Here's how the part is built. I have some questions about the finished solid (model axes, mm). Face numbers are marked on the shaded views. A direction names the side the tool comes from. Round coordinates to 2 decimals unless told otherwise and drop trailing zeros. Order: outer loops, then holes, each group sorted by start corner. A loop starts at its lowest first (then second) coordinate and runs counter-clockwise, first axis right, second up. Notation, with made-up numbers: (18.25, 35.25) -> (66.25, 35.25) arc R29 ccw to (66.25, 74.25) -> close; hole circle Ø7 at (48.25, 61). An arc over 180 degrees is marked (long way). Answer in a Markdown table with one row per item.
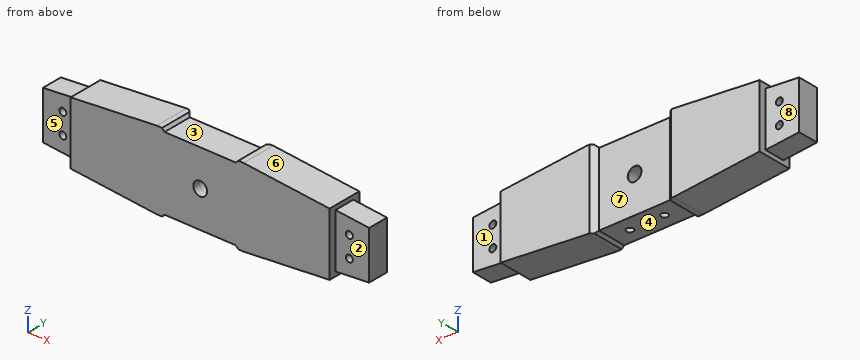
```python
from build123d import *

# Parameters (mm, degrees)
SKETCH1_R                = 4
BOSS_EXTRUDE1_DEPTH      = 12
SKETCH2_R                = 4
BOSS_EXTRUDE2_DEPTH      = 4
BOSS_EXTRUDE2_DEPTH_BACK = 16
CUT_EXTRUDE1_DEPTH       = 1
CUT_EXTRUDE1_DEPTH_BACK  = 46
SKETCH6_R                = 2.05
CUT_EXTRUDE3_DEPTH       = 6.5
SKETCH7_R                = 2
CUT_EXTRUDE4_DEPTH       = 17
CUT_EXTRUDE5_DEPTH       = 1
CUT_EXTRUDE5_DEPTH_BACK  = 21
CUT_EXTRUDE6_DEPTH       = 17


with BuildPart() as part:
    # Sketch1 → Boss-Extrude1 (new body)
    with BuildSketch(Plane(origin=(0, 0, 0), x_dir=(1, 0, 0), z_dir=(0, 1, 0))):
        Polygon((25, 20), (-25, 20), (-95, 13.834935185), (-95, -13.834935185), (-25, -20), (25, -20), (95, -13.834935185), (95, 13.834935185), align=None)
        Circle(SKETCH1_R, mode=Mode.SUBTRACT)
    extrude(amount=BOSS_EXTRUDE1_DEPTH)

    # Sketch2 → Boss-Extrude2 (add, two sides)
    with BuildSketch(Plane(origin=(0, 12, 0), x_dir=(1, 0, 0), z_dir=(0, 1, 0))) as boss_extrude2_sk:
        Polygon((-25, 20), (-75, 15.596382275), (-75, -15.596382275), (-25, -20), (25, -20), (75, -15.596382275), (75, 15.596382275), (25, 20), align=None)
        Circle(SKETCH2_R, mode=Mode.SUBTRACT)
        Polygon((-25, -20), (-75, -15.596382275), (-75, -18.10605947), (-25.109877781, -22.5), (25.109877781, -22.5), (75, -18.10605947), (75, -15.596382275), (25, -20), align=None)
        Polygon((-25.109877781, 22.5), (-75, 18.10605947), (-75, 15.596382275), (-25, 20), (25, 20), (75, 15.596382275), (75, 18.10605947), (25.109877781, 22.5), align=None)
    extrude(amount=BOSS_EXTRUDE2_DEPTH)
    extrude(boss_extrude2_sk.sketch, amount=-BOSS_EXTRUDE2_DEPTH_BACK)

    # Sketch3 → Cut-Extrude1 (cut, two sides)
    with BuildSketch(Plane.XY.offset(22.5)) as cut_extrude1_sk:
        Polygon((23.609877781, 16), (-23.609877781, 16), (-20.609877781, 13), (20.609877781, 13), align=None)
    extrude(amount=CUT_EXTRUDE1_DEPTH, mode=Mode.SUBTRACT)
    extrude(cut_extrude1_sk.sketch, amount=-CUT_EXTRUDE1_DEPTH_BACK, mode=Mode.SUBTRACT)

    # Sketch6 → Cut-Extrude3 (cut)
    with BuildSketch(Plane(origin=(0, 0, -22.5), x_dir=(-1, 0, 0), z_dir=(0, 0, -1))):
        with Locations((-10, 4.5)):
            Circle(SKETCH6_R)
        with Locations((10, 4.5)):
            Circle(SKETCH6_R)
    extrude(amount=-CUT_EXTRUDE3_DEPTH, mode=Mode.SUBTRACT)

    # Sketch7 → Cut-Extrude4 (cut, through all)
    with BuildSketch(Plane.XZ):
        with Locations((-83, -6)):
            Circle(SKETCH7_R)
        with Locations((-83, 6)):
            Circle(SKETCH7_R)
        with Locations((83, 6)):
            Circle(SKETCH7_R)
        with Locations((83, -6)):
            Circle(SKETCH7_R)
    extrude(amount=-CUT_EXTRUDE4_DEPTH, mode=Mode.SUBTRACT)

    # Sketch8 → Cut-Extrude5 (cut, two sides)
    with BuildSketch(Plane.XZ.offset(4)) as cut_extrude5_sk:
        Polygon((-22.109877781, -22.5), (-20.609877781, -21), (20.609877781, -21), (22.109877781, -22.5), align=None)
        Polygon((-22.109877781, 22.5), (22.109877781, 22.5), (20.609877781, 21), (-20.609877781, 21), align=None)
    extrude(amount=CUT_EXTRUDE5_DEPTH, mode=Mode.SUBTRACT)
    extrude(cut_extrude5_sk.sketch, amount=-CUT_EXTRUDE5_DEPTH_BACK, mode=Mode.SUBTRACT)

    # Sketch9 → Cut-Extrude6 (cut, through all)
    with BuildSketch(Plane(origin=(0, 12, 0), x_dir=(1, 0, 0), z_dir=(0, 1, 0))):
        Polygon((-94.5, 13.878971362), (-94.5, -13.878971362), (-95, -13.834935185), (-95, 13.834935185), align=None)
        Polygon((94.5, 13.878971362), (94.5, -13.878971362), (95, -13.834935185), (95, 13.834935185), align=None)
    extrude(amount=-CUT_EXTRUDE6_DEPTH, mode=Mode.SUBTRACT)


solid = part.part
```
1. Suppose I cut it at A-A on z = -6. Write out the boundary of the cut face in (x, y).
Numbers:
| item | result |
|---|---|
| outline | (-94.5, 0) -> (-85, 0) -> (-85, 12) -> (-94.5, 12) -> close; (-81, 0) -> (-75, 0) -> (-75, -4) -> (75, -4) -> (75, 0) -> (81, 0) -> (81, 12) -> (75, 12) -> (75, 16) -> (23.61, 16) -> (20.61, 13) -> (-20.61, 13) -> (-23.61, 16) -> (-75, 16) -> (-75, 12) -> (-81, 12) -> close; (85, 0) -> (94.5, 0) -> (94.5, 12) -> (85, 12) -> close |
2. Suppose I cut it at C-C on z = 10. Write out the boundary of the cut face in (x, y), then the cut area to 3 significant figures.
Numbers:
| item | result |
|---|---|
| outline | (-94.5, 0) -> (-75, 0) -> (-75, -4) -> (75, -4) -> (75, 0) -> (94.5, 0) -> (94.5, 12) -> (75, 12) -> (75, 16) -> (23.61, 16) -> (20.61, 13) -> (-20.61, 13) -> (-23.61, 16) -> (-75, 16) -> (-75, 12) -> (-94.5, 12) -> close |
| area | 3,340 mm2 |
3. Suppose I cut it at D-D on x = -83. Write out the boundary of the cut face in (y, z), then the cut area to 3 significant figures.
Numbers:
| item | result |
|---|---|
| outline | (0, -14.89) -> (12, -14.89) -> (12, -8) -> (0, -8) -> close; (0, -4) -> (12, -4) -> (12, 4) -> (0, 4) -> close; (0, 8) -> (12, 8) -> (12, 14.89) -> (0, 14.89) -> close |
| area | 261 mm2 |
4. We'd pull the mould along X, two halves only. Please class the marked faces 6, 7 and 8: released by +X, released by -X, zero draft, split by the parting line, or undercut.
Numbers:
| item | result |
|---|---|
| face 6 | released by +X |
| face 7 | undercut |
| face 8 | zero draft |
5. Please list where these lines run through material, in increasing order: line 1 along Y through (x, z) = (10, -19.3); line 2 along Z through (x, y) = (0, -2.95); line 3 along X through (y, z) = (-2.9, 0).
Numbers:
| item | result |
|---|---|
| line 1 | y = -4 to 2.45, 6.55 to 13 |
| line 2 | z = -21 to -4, 4 to 21 |
| line 3 | x = -75 to -4, 4 to 75 |
6. Suppose I cut it at B-B on x = 0. Write out the boundary of the cut face in (y, z), then the cut area to 3 significant figures.
Numbers:
| item | result |
|---|---|
| outline | (-4, -21) -> (13, -21) -> (13, -4) -> (-4, -4) -> close; (-4, 4) -> (13, 4) -> (13, 21) -> (-4, 21) -> close |
| area | 578 mm2 |
7. For the marked faces 1, 2, 3, 4 and 5, which set-ups out of +Z, -Z, +X, -X, +Y, -Y let a thin tool reach every point of the face, with its end or its side?
Numbers:
| item | result |
|---|---|
| face 1 | +Z, -Z, +X, +Y |
| face 2 | +Z, -Z, +X, -Y |
| face 3 | +Z, +Y, -Y |
| face 4 | -Z, +Y, -Y |
| face 5 | +Z, -Z, -X, -Y |
8. For pin 1 Ø6 at (x, z) = (84, 1.5) entering from -Y; pin 2 Ø4 at (x, y) = (45.5, 6) entering from -Z; pin 3 Ø2.5 at (x, y) = (-10, 4.5) entering from +Z, each with a flat end and sliding along its axis, tell me the tip position at first contact or that it passes through.
Numbers:
| item | result |
|---|---|
| pin 1 | stops at y = 0 |
| pin 2 | stops at z = -20.88 |
| pin 3 | stops at z = 21 |
